Verification items for this drawing (mm, ordinates from the low corner). Round coordinates to 2 decimals unless told otherwise and drop trailing zeros. Loops run counter-clockwise (first coordinate to the right, second up) from the corner with the lowest first, then second, coordinate; pieces in that order, holes last. Notation, with made-up numbers: (35.25, 57.25) -> (89.25, 57.25) arc R22 ccw to (89.25, 89.25) -> close; hole circle Ø9 at (81, -32). An arc over 180 degrees is marked (long way). One line per item, written item: value. Start each with the question number.
1. Cross-section at D-D on x = 1.25. Record the cut outline in (y, z).
2. Material ranges on L1, parallel to Z at x = 7.75, y = 0.25; L2, parallel to Z at x = 6.5, y = 0.15 (1 decimal); L3, parallel to X at y = 1, z = 30.5 (1 decimal), recorded low to high.
3. Go/stop test with flat-tipped pins: pin 1 (5 mm diameter, centred on x = 7.54, z = 4.76, fed in from -Y); pin 2 (3.5 mm diameter, centred on x = 7.54, z = 30.16, fed in from -Y). Record where each tip stops, or that it passes through.
4. Cross-section at C-C on z = 33.5. Record the cut outline in (x, y).
5. Cross-section at A-A on y = 1. Count the separate pieces of the cut face and the enclosed holes in it.
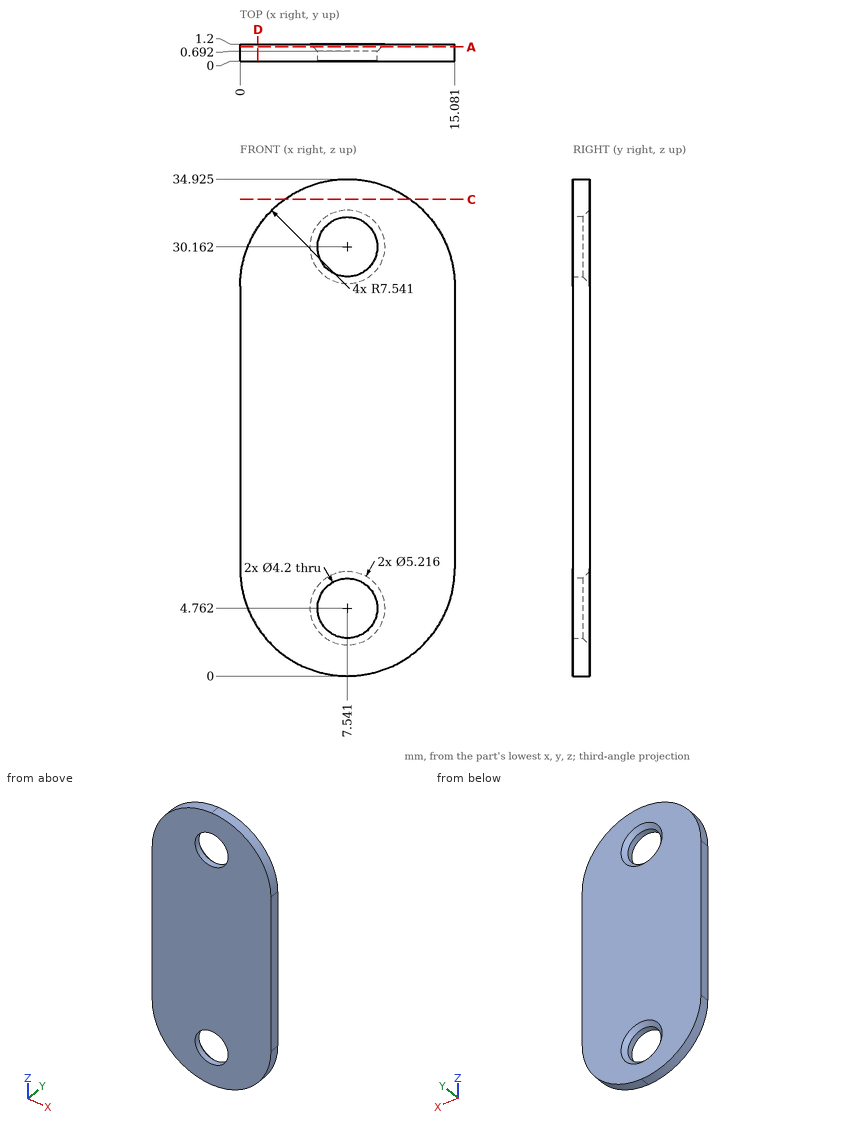
Taken from the geometry:
1. outline: (0, 3.38) -> (1.2, 3.38) -> (1.2, 31.54) -> (0, 31.54) -> close
2. L1: z = 0 to 2.67, 6.85 to 28.07, 32.25 to 34.92
2. L2: z = 0.1 to 2.9, 6.6 to 28.3, 32 to 34.9
2. L3: x = 0.7 to 5.2, 9.9 to 14.4
3. pin 1: stops at y = 0
3. pin 2: passes through
4. outline: (3.13, 0) -> (11.95, 0) -> (11.95, 1.2) -> (3.13, 1.2) -> close
5. separate pieces: 1
5. enclosed holes: 2
